Check sheet for the modelled part. Datum: model origin and axes. Units: mm. Face numbers are marked on the shaded views. A direction names the side the tool comes from. Round coordinates to 2 decimals unless told otherwise and drop trailing zeros. Write each loop counter-clockwise with the first axis right and the second up, starting at its lowest first coordinate (ties: lowest second). Pieces come first, ordered by that corner, then holes.
from build123d import *

# Parameters (mm, degrees)
F0_W = 3
F0_H = 3.5
F2_R = 5.99999


# Not quite as in the source:
# - a fillet or chamfer is up to 0.001 mm smaller than in the source, because OpenCascade refuses the exact size


with BuildPart() as f1:
    # F0 (on Right) → F1 (revolve)
    with BuildSketch(Plane.YZ):
        with Locations((-36.5, 14.25)):
            Rectangle(F0_W, F0_H)
        Polygon((-18, 12.5), (-18, 20), (-35, 20), (-35, 16), (-35, 12.5), align=None)
        Polygon((-6, 12.5), (-6, 31), (-18, 31), (-18, 20), (-18, 12.5), align=None)
        with BuildLine():
            Line((6, 12.5), (6, 31))
            ThreePointArc((6, 31), (0, 25), (-6, 31))
            Line((-6, 31), (-6, 12.5))
            Line((-6, 12.5), (6, 12.5))
        make_face()
        Polygon((50, 31), (6, 31), (6, 12.5), (20, 12.5), (20, 16), (28, 16), (28, 20.5), (35, 20.5), (35, 14), (38, 14), (38, 16), (48.5, 16), (48.5, 25), (50, 25), align=None)
    revolve(axis=Axis((0, 8.8457800448, 0), (0, 1, 0)))

    # F2 (radius 6 in the source; OpenCascade refuses exactly that, so slightly less here)
    f2_edges = [f1.edges().sort_by_distance(p)[0] for p in [
        (0, 50, -31),
    ]]
    fillet(f2_edges, radius=F2_R)


solid = f1.part
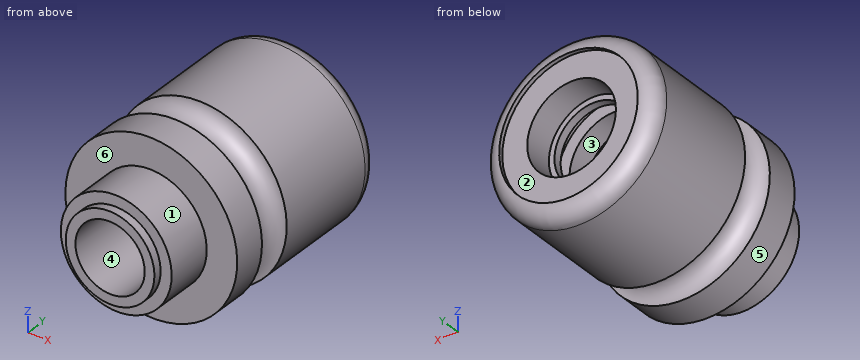
1. Sectioned sample at A-A, the plane y = 30. Enter the section's corners in (x, z), plus the area to 3 significant figures.
2. Go/stop test with flat-tipped pins: pin 1 (3 mm diameter, centred on x = 10, y = -11.5, fed in from +Z); pin 2 (22.5 mm diameter, centred on x = 0, z = 0, fed in from +Y); pin 3 (15 mm diameter, centred on x = -1, z = -8, fed in from +Y); pin 4 (3 mm diameter, centred on x = -10, y = -28, fed in from +Z). Record where each tip stops, or that it passes through.
3. Sectioned sample at B-B, the plane y = -12. Enter the section's corners in (x, z), plus the area to 3 significant figures.
4. Release check for a two-part mould opening along Z. For the marked faces 4, 5 and 6 record: released by +Z, released by -Z, zero draft, split by the parting line, or undercut.
5. Scan lines: line 1 along Y through (x, z) = (-19, -1.5); line 2 along Y through (x, z) = (-15, 1); line 3 along Y through (x, z) = (4, -20.5). Record each from-to range of solid material in increasing order.
6. Set-up check for the marked faces 1, 2 and 3: record each of +Z, -Z, +X, -X, +Y, -Y from which the full face is reachable in a straight line by a thin tool's end or side.
Computed values:
1. outline: circle Ø62 at (0, 0); hole circle Ø41 at (0, 0)
1. area: 1,700 mm2
2. pin 1: stops at z = 29.81
2. pin 2: passes through
2. pin 3: stops at y = 38
2. pin 4: stops at z = 18.1
3. outline: circle Ø62 at (0, 0); hole circle Ø25 at (0, 0)
3. area: 2,530 mm2
4. face 4: undercut
4. face 5: split by the parting line
4. face 6: zero draft
5. line 1: y = -35 to 28, 35 to 48.5
5. line 2: y = -38 to 20, 35 to 38
5. line 3: y = -18 to 48.5
6. face 1: -Y
6. face 2: +Y
6. face 3: none
